CAD build for the part. Positions are in the model's coordinates, mm. Face numbers are marked on the shaded views. A direction names the side the tool comes from. Round coordinates to 2 decimals unless told otherwise and drop trailing zeros. Order: outer loops, then holes, each group sorted by start corner. A loop starts at its lowest first (then second) coordinate and runs counter-clockwise, first axis right, second up. Notation, with made-up numbers: M -29,15.5 L 15,15.5 A13 ccw 15,22.5 Z; hole C 70,79.5 d3. An arc over 180 degrees is marked long. Put each result on its own line as item: value.
```python
from build123d import *

# Parameters (mm, degrees)
F1_DEPTH = 12.5


with BuildPart() as f1:
    # F0 (on Right) → F1 (new body, symmetric)
    with BuildSketch(Plane.YZ):
        with BuildLine():
            Line((0, 180), (0, 0))
            Line((0, 0), (80, 0))
            Line((80, 0), (80, 210))
            ThreePointArc((80, 210), (68.284271, 238.284271), (40, 250))
            Line((40, 250), (-60, 250))
            Line((-60, 250), (-60, 220))
            Line((-60, 220), (-40, 220))
            ThreePointArc((-40, 220), (-11.715729, 208.284271), (0, 180))
        make_face()
    extrude(amount=F1_DEPTH, both=True)


solid = f1.part
```
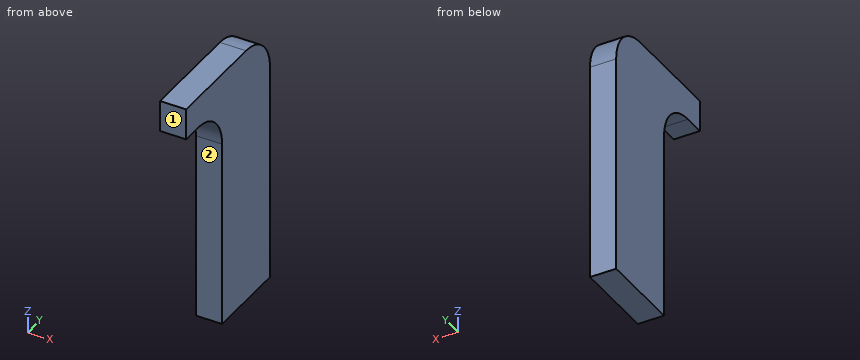
Item 1: Probe line 1 along Y through (x, z) = (4, 15.5); line 2 along Z through (x, y) = (7, -44); line 3 along Z through (x, y) = (8, -34.5). List the from-to ranges inside material, lowest first. Write a range as [from, to].
Answers below:
line 1: [0, 80]
line 2: [220, 250]
line 3: [219.62, 250]
Item 2: Band-saw the part on B-B on z = 26.5. Give the cut face in (x, y), and give its area (3 significant figures).
Answers below:
outline: M -12.5,0 L 12.5,0 L 12.5,80 L -12.5,80 Z
area: 2,000 mm²
Item 3: Tool access for the marked faces 1 and 2: list every direction of +Z, -Z, +X, -X, +Y, -Y with a clear straight run to the whole face (end or side of a thin tool).
Answers below:
face 1: +Z, -Z, +X, -X, -Y
face 2: -Z, +X, -X, -Y
Item 4: Band-saw the part on A-A on x = -0.5. Give the cut face in (y, z), and give its area (3 significant figures).
Answers below:
outline: M -60,220 L -40,220 A40 cw 0,180 L 0,0 L 80,0 L 80,210 A40 ccw 40,250 L -60,250 Z
area: 21,800 mm²
Item 5: Band-saw the part on C-C on y = -46.5. Give the cut face in (x, z), and give its area (3 significant figures).
Answers below:
outline: M -12.5,220 L 12.5,220 L 12.5,250 L -12.5,250 Z
area: 750 mm²
Item 6: Pin check, flat tips, straight feed: P1, Ø2, axis at x = -7.5, z = 165.5, coming from the -Y side; P2, Ø10, axis at x = -0.5, y = -45.5, coming from the -Z side. Stop position of each tip, or through.
Answers below:
P1: y = 0
P2: z = 220
